from build123d import *

# Parameters (mm, degrees)
SKETCH1_W           = 30
SKETCH1_H           = 12
BOSS_EXTRUDE1_DEPTH = 3
SKETCH2_W           = 3
SKETCH2_H           = 12
BOSS_EXTRUDE2_DEPTH = 40
FILLET1_R           = 3
FILLET2_R           = 3
SKETCH3_R           = 4
CUT_EXTRUDE1_DEPTH  = 40
SKETCH4_R           = 3
CUT_EXTRUDE3_DEPTH  = 49.631265663
FILLET3_R           = 6
FILLET4_R           = 6


with BuildPart() as part:
    # Sketch1 → Boss-Extrude1 (new body)
    with BuildSketch(Plane(origin=(0, 0, 0), x_dir=(1, 0, 0), z_dir=(0, 1, 0))):
        Rectangle(SKETCH1_W, SKETCH1_H)
    extrude(amount=BOSS_EXTRUDE1_DEPTH)

    # Sketch2 → Boss-Extrude2 (add)
    with BuildSketch(Plane.XZ):
        with Locations((13.5, 0)):
            Rectangle(SKETCH2_W, SKETCH2_H)
    extrude(amount=BOSS_EXTRUDE2_DEPTH)

    # Fillet1
    fillet1_edges = [part.edges().sort_by_distance(p)[0] for p in [
        (15, 3, 0),
    ]]
    fillet(fillet1_edges, radius=FILLET1_R)

    # Fillet2
    fillet2_edges = [part.edges().sort_by_distance(p)[0] for p in [
        (12, 0, 0),
    ]]
    fillet(fillet2_edges, radius=FILLET2_R)

    # Sketch3 → Cut-Extrude1 (cut)
    with BuildSketch(Plane(origin=(0, 3, 0), x_dir=(1, 0, 0), z_dir=(0, 1, 0))):
        with Locations(Location((-2.5, 0, 0), (0, 0, 270))):
            Circle(SKETCH3_R)
    extrude(amount=-CUT_EXTRUDE1_DEPTH, mode=Mode.SUBTRACT)

    # Sketch4 → Cut-Extrude3 (cut, through all)
    with BuildSketch(Plane.ZY.offset(-12)):
        with Locations((0, -15)):
            Circle(SKETCH4_R)
        with Locations((0, -30)):
            Circle(SKETCH4_R)
    extrude(amount=-CUT_EXTRUDE3_DEPTH, mode=Mode.SUBTRACT)

    # Fillet3
    fillet3_edges = [part.edges().sort_by_distance(p)[0] for p in [
        (-15, 1.5, -6),
        (-15, 1.5, 6),
    ]]
    fillet(fillet3_edges, radius=FILLET3_R - 0.0001)  # a hair under: the kernel refuses the full size

    # Fillet4
    fillet4_edges = [part.edges().sort_by_distance(p)[0] for p in [
        (13.5, -40, 6),
        (13.5, -40, -6),
    ]]
    fillet(fillet4_edges, radius=FILLET4_R - 0.0001)  # a hair under: the kernel refuses the full size


solid = part.part
Verification items for the finished model (mm, model axes). A direction names the side the tool comes from. Give positions to 0.01 mm unless a question says otherwise; leave off trailing zeros. Loops run counter-clockwise (first coordinate to the right, second up) from the corner with the lowest first, then second, coordinate; pieces in that order, holes last. Notation, with made-up numbers: (-6, 36) - (22, 36) arc R24 cw to (22, 56) - close; hole circle Ø11 at (1, 57). An arc over 180 degrees is marked (long way). Write item = value, one per line. Start each with the question number.
Q1. Mould release check, pull along Z, two halves, no side actions. Record for faces 3 (the face through (13, -10, -6)), 4 (the face through (-3.2, 0, -4.1)), 5 (the face through (13.521, -38.196, 4.289)), 6 (the face through (13.48, -17.93, -0.65)): released by +Z, released by -Z, zero draft, split by the parting line, or undercut.
Q2. Tool access check on faces 1 (the face through (12, -21, 0)), 2 (the face through (-13.289, 1.521, -4.196)). Record the directions out of +Z, -Z, +X, -X, +Y, -Y that give a thin tool (end or side, any length) a straight path to the whole face; none if there is none.
Q3. Cross-section at D-D, the plane x = 3.25. Enter the section's corners in (y, z), and give its area (3 significant figures).
Q4. Cross-section at A-A, the plane y = -30. Enter the section's corners in (x, z).
Q5. Cross-section at C-C, the plane z = -2.5. Enter the section's corners in (x, y), and give its area (3 significant figures).
Q6. Cross-section at B-B, the plane z = 3.5. Enter the section's corners in (x, y), and give its area (3 significant figures).
Q7. Thickness scan on line 1 (Y direction, x = 13.2, z = 0); line 2 (Y direction, x = 12.9, z = 0); line 3 (X direction, y = -18.5, z = -2). Record the ranges inside material, lowest first.
Q8. Depth check by flat-ended pin: P1, Ø3, axis at y = -12.5, z = -1, coming from the +X side; P2, Ø2, axis at x = 12, z = -3, coming from the -Y side; P3, Ø5, axis at x = -2.5, z = 0, coming from the +Y side; P4, Ø6, axis at x = -11, z = 2.5, coming from the -Y side. Enter the tip coordinate at first touch or a pass-through.
Answer key:
q1.face_3 = released by -Z
q1.face_4 = zero draft
q1.face_5 = released by +Z
q1.face_6 = undercut
q2.face_1 = +Z, -Z, -X, -Y
q2.face_2 = -Z, -X, +Y, -Y
q3.outline = (0, -6) - (3, -6) - (3, 6) - (0, 6) - close
q3.area = 36.0 mm^2
q4.outline = (12, -6) - (15, -6) - (15, -3) - (12, -3) - close; (12, 3) - (15, 3) - (15, 6) - (12, 6) - close
q5.outline = (-14.45, 0) - (-5.62, 0) - (-5.62, 3) - (-14.45, 3) - close; (0.62, 0) - (9, 0) arc R3 cw to (12, -3) - (12, -13.34) - (15, -13.34) - (15, 0) arc R3 ccw to (12, 3) - (0.62, 3) - close; (12, -39.45) - (15, -39.45) - (15, -31.66) - (12, -31.66) - close; (12, -28.34) - (15, -28.34) - (15, -16.66) - (12, -16.66) - close
q5.area = 168 mm^2
q6.outline = (-13.87, 0) - (-4.44, 0) - (-4.44, 3) - (-13.87, 3) - close; (-0.56, 0) - (9, 0) arc R3 cw to (12, -3) - (12, -38.87) - (15, -38.87) - (15, 0) arc R3 ccw to (12, 3) - (-0.56, 3) - close
q6.area = 192 mm^2
q7.line_1 = -40 to -33, -27 to -18, -12 to 2.75
q7.line_2 = -40 to -33, -27 to -18, -12 to 2.86
q7.line_3 = 12 to 15
q8.P1 = 15
q8.P2 = -39.66
q8.P3 = through
q8.P4 = 0
